For this review, take the finished solid that the model builds, in its own axes (mm). Face numbers are marked on the shaded views. Round coordinates to 2 decimals unless told otherwise and drop trailing zeros. Order: outer loops, then holes, each group sorted by start corner. A loop starts at its lowest first (then second) coordinate and runs counter-clockwise, first axis right, second up.
```python
from build123d import *

# Parameters (mm, degrees)
SKETCH_1_R             = 12
EXTRUDE_1_DEPTH        = 10
CHAMFER_1_SIZE         = 0.5
HOLE_WIZARD_M8_1_D     = 6.8
HOLE_WIZARD_M8_1_DEPTH = 17.707073895
HOLE_WIZARD_M8_1_TIP   = 2.042926105
F_3_0MM_1_D            = 3
F_3_0MM_1_DEPTH        = 18.848709071
F_3_0MM_1_TIP          = 0.901290929


with BuildPart() as part:
    # 草图1 → 凸台-拉伸1 (new body)
    with BuildSketch(Plane.XY):
        Circle(SKETCH_1_R)
    extrude(amount=EXTRUDE_1_DEPTH)

    # 倒角1
    chamfer_1_edges = [part.edges().sort_by_distance(p)[0] for p in [
        (-12, 0, 0),
        (-12, 0, 10),
    ]]
    chamfer(chamfer_1_edges, length=CHAMFER_1_SIZE)

    # M8 螺纹孔1
    with Locations(Plane.XY.offset(10)):
        with Locations((0, 0)):
            Hole(HOLE_WIZARD_M8_1_D / 2, depth=HOLE_WIZARD_M8_1_DEPTH)
            with Locations((0, 0, -(HOLE_WIZARD_M8_1_DEPTH + HOLE_WIZARD_M8_1_TIP / 2))):  # 118° drill point
                Cone(0, HOLE_WIZARD_M8_1_D / 2, HOLE_WIZARD_M8_1_TIP, mode=Mode.SUBTRACT)

    # Ø3.0mm 暗销孔1
    with Locations(Plane.XY.offset(10)):
        with Locations((0, -8), (0, 8)):
            Hole(F_3_0MM_1_D / 2, depth=F_3_0MM_1_DEPTH)
            with Locations((0, 0, -(F_3_0MM_1_DEPTH + F_3_0MM_1_TIP / 2))):  # 118° drill point
                Cone(0, F_3_0MM_1_D / 2, F_3_0MM_1_TIP, mode=Mode.SUBTRACT)


solid = part.part
```
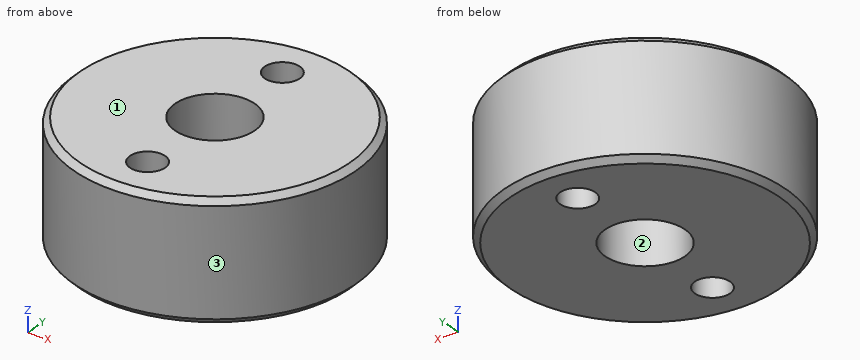
Q1. Take a section at C-C, the plane z = 7.25. State the section outline as (x, y) points, plus the area to 3 significant figures.
Q2. Take a section at B-B, the plane y = 0. State the section outline as (x, z) points, plus the area to 4 significant figures.
Q3. Wall thickness on line 1 (Y direction, x = 0, z = 3); line 2 (X direction, y = -1.75, z = 7.75); line 3 (X direction, y = -9, z = 6.75): over which ranges is each line inside the solid? List them lowest first.
Q4. Mouldability with a two-part tool opening along X and no side actions: class the marked faces 1, 2 and 3 as +X half, -X half, draft (parallel to the pull), parting line (faces both ways), or undercut.
Q5. Take a section at A-A, the plane x = 0. State the section outline as (y, z) points.
Q6. Clearance check with flat-ended pins moving along their axes: pin 1 (1.5 mm diameter, centred on y = -3, z = 3.5, fed in from +X); pin 2 (6 mm diameter, centred on y = 9.5, z = 4, fed in from -X); pin 3 (1.8 mm diameter, centred on x = 0, y = 8, fed in from +Z); pin 4 (4 mm diameter, centred on x = 8.5, z = 7, fed in from +Y). State where each tip first meets the part, or that it passes through.
Working result:
1. outline: circle Ø24 at (0, 0); hole circle Ø6.8 at (0, 0); hole circle Ø3 at (0, -8); hole circle Ø3 at (0, 8)
1. area: 402 mm2
2. outline: (-12, 0.5) - (-11.5, 0) - (-3.4, 0) - (-3.4, 10) - (-11.5, 10) - (-12, 9.5) - close; (3.4, 0) - (11.5, 0) - (12, 0.5) - (12, 9.5) - (11.5, 10) - (3.4, 10) - close
2. area: 171.5 mm2
3. line 1: y = -12 to -9.5, -6.5 to -3.4, 3.4 to 6.5, 9.5 to 12
3. line 2: x = -11.87 to -2.92, 2.92 to 11.87
3. line 3: x = -7.94 to -1.12, 1.12 to 7.94
4. face 1: draft
4. face 2: undercut
4. face 3: parting line
5. outline: (-12, 0.5) - (-11.5, 0) - (-9.5, 0) - (-9.5, 10) - (-11.5, 10) - (-12, 9.5) - close; (-6.5, 0) - (-3.4, 0) - (-3.4, 10) - (-6.5, 10) - close; (3.4, 0) - (6.5, 0) - (6.5, 10) - (3.4, 10) - close; (9.5, 0) - (11.5, 0) - (12, 0.5) - (12, 9.5) - (11.5, 10) - (9.5, 10) - close
6. pin 1: stops at x = 11.79
6. pin 2: stops at x = -10.09
6. pin 3: passes through
6. pin 4: stops at y = 10.09
